```python
from build123d import *

# Parameters (mm, degrees)
SKETCH_1_W                   = 100
SKETCH_1_H                   = 100
EXTRUDE_1_DEPTH              = 5
CUT_EXTRUDE_1_REACH          = 72.887
SKETCH_2_W                   = 12.5
SKETCH_2_H                   = 22.4
HOLE_WIZARD_M2_3_D           = 2.4
HOLE_WIZARD_M2_3_CBORE_D     = 4.4
HOLE_WIZARD_M2_3_CBORE_DEPTH = 2
SKETCH_9_W                   = 25
SKETCH_9_H                   = 6.5
SKETCH_9_W_2                 = 6.5
SKETCH_9_H_2                 = 42.2
EXTRUDE_4_DEPTH              = 20
HOLE_WIZARD_M2_4_D           = 2.4
HOLE_WIZARD_M2_4_CBORE_D     = 4.4
HOLE_WIZARD_M2_4_CBORE_DEPTH = 2
SKETCH_12_W                  = 42
SKETCH_12_H                  = 5
CUT_EXTRUDE_2_DEPTH          = 10
CUT_EXTRUDE_3_DEPTH          = 91.444513377


with BuildPart() as part:
    # 草图1 → 凸台-拉伸1 (new body)
    with BuildSketch(Plane(origin=(0, 0, 0), x_dir=(1, 0, 0), z_dir=(0, 1, 0))):
        Rectangle(SKETCH_1_W, SKETCH_1_H)
    extrude(amount=EXTRUDE_1_DEPTH)

    # 草图2 → 切除-拉伸1 (cut, up to next)
    with BuildSketch(Plane(origin=(0, 5, 0), x_dir=(1, 0, 0), z_dir=(0, 1, 0)), mode=Mode.PRIVATE) as cut_extrude_1_sk1:
        with Locations((-43.75, 32.3)):
            Rectangle(SKETCH_2_W, SKETCH_2_H)
    cut_extrude_1_tool1 = extrude(cut_extrude_1_sk1.sketch, amount=-CUT_EXTRUDE_1_REACH, mode=Mode.PRIVATE) & part.part
    # 草图2 → 切除-拉伸1 (cut, up to next)
    with BuildSketch(Plane(origin=(0, 5, 0), x_dir=(1, 0, 0), z_dir=(0, 1, 0)), mode=Mode.PRIVATE) as cut_extrude_1_sk2:
        with Locations((43.75, 32.3)):
            Rectangle(SKETCH_2_W, SKETCH_2_H)
    cut_extrude_1_tool2 = extrude(cut_extrude_1_sk2.sketch, amount=-CUT_EXTRUDE_1_REACH, mode=Mode.PRIVATE) & part.part
    # 草图2 → 切除-拉伸1 (cut, up to next)
    with BuildSketch(Plane(origin=(0, 5, 0), x_dir=(1, 0, 0), z_dir=(0, 1, 0)), mode=Mode.PRIVATE) as cut_extrude_1_sk3:
        with Locations((43.75, -32.3)):
            Rectangle(SKETCH_2_W, SKETCH_2_H)
    cut_extrude_1_tool3 = extrude(cut_extrude_1_sk3.sketch, amount=-CUT_EXTRUDE_1_REACH, mode=Mode.PRIVATE) & part.part
    # 草图2 → 切除-拉伸1 (cut, up to next)
    with BuildSketch(Plane(origin=(0, 5, 0), x_dir=(1, 0, 0), z_dir=(0, 1, 0)), mode=Mode.PRIVATE) as cut_extrude_1_sk4:
        with Locations((-43.75, -32.3)):
            Rectangle(SKETCH_2_W, SKETCH_2_H)
    cut_extrude_1_tool4 = extrude(cut_extrude_1_sk4.sketch, amount=-CUT_EXTRUDE_1_REACH, mode=Mode.PRIVATE) & part.part
    add(cut_extrude_1_tool1.solids().sort_by_distance((-43.75, 5, -32.3))[0], mode=Mode.SUBTRACT)
    add(cut_extrude_1_tool2.solids().sort_by_distance((43.75, 5, -32.3))[0], mode=Mode.SUBTRACT)
    add(cut_extrude_1_tool3.solids().sort_by_distance((43.75, 5, 32.3))[0], mode=Mode.SUBTRACT)
    add(cut_extrude_1_tool4.solids().sort_by_distance((-43.75, 5, 32.3))[0], mode=Mode.SUBTRACT)

    # M2 凹头盖螺钉的柱形沉头孔3 (through all)
    with Locations(Plane(origin=(-43.75, 5, -46.15), x_dir=(0, 0, 1), z_dir=(0, 1, 0))):
        with Locations((0, 0), (0, 87.5), (27.7, 87.5), (27.7, 0), (64.6, 0), (92.3, 0), (64.6, 87.5), (92.3, 87.5)):
            CounterBoreHole(HOLE_WIZARD_M2_3_D / 2, HOLE_WIZARD_M2_3_CBORE_D / 2, HOLE_WIZARD_M2_3_CBORE_DEPTH)

    # 草图9 → 凸台-拉伸4 (add)
    with BuildSketch(Plane(origin=(0, 5, 0), x_dir=(1, 0, 0), z_dir=(0, 1, 0))):
        with Locations((0, 46.75)):
            Rectangle(SKETCH_9_W, SKETCH_9_H)
        with Locations((0, -46.75)):
            Rectangle(SKETCH_9_W, SKETCH_9_H)
        with Locations((-34.25, 0)):
            Rectangle(SKETCH_9_W_2, SKETCH_9_H_2)
        with Locations((34.25, 0)):
            Rectangle(SKETCH_9_W_2, SKETCH_9_H_2)
    extrude(amount=EXTRUDE_4_DEPTH)

    # M2 凹头盖螺钉的柱形沉头孔4 (through all)
    with Locations(Plane(origin=(-17, 5, -25), x_dir=(0, 0, 1), z_dir=(0, 1, 0))):
        with Locations((0, 0), (0, 34), (50, 0), (50, 34)):
            CounterBoreHole(HOLE_WIZARD_M2_4_D / 2, HOLE_WIZARD_M2_4_CBORE_D / 2, HOLE_WIZARD_M2_4_CBORE_DEPTH)

    # 草图12 → 切除-拉伸2 (cut)
    with BuildSketch(Plane(origin=(0, 5, 0), x_dir=(1, 0, 0), z_dir=(0, 1, 0))):
        with Locations((0, 36.5)):
            Rectangle(SKETCH_12_W, SKETCH_12_H)
        with Locations((0, -36.5)):
            Rectangle(SKETCH_12_W, SKETCH_12_H)
    extrude(amount=-CUT_EXTRUDE_2_DEPTH, mode=Mode.SUBTRACT)

    # 草图15 → 切除-拉伸3 (cut, through all)
    with BuildSketch(Plane.XY.offset(21.1)):
        Polygon((-37.5, 25), (-37.5, 22), (-35.5, 22), align=None)
        Polygon((-31, 25), (-31, 22), (-33, 22), align=None)
        Polygon((37.5, 25), (37.5, 22), (35.5, 22), align=None)
        Polygon((31, 22), (33, 22), (31, 25), align=None)
    extrude(amount=-CUT_EXTRUDE_3_DEPTH, mode=Mode.SUBTRACT)


solid = part.part
```
CAD build for the part. Positions are in the model's coordinates, mm. A direction names the side the tool comes from. Coordinates: 2 decimals unless noted, no trailing zeros. Order: outer loops, then holes, each group sorted by start corner. A loop starts at its lowest first (then second) coordinate and runs counter-clockwise, first axis right, second up. Notation, with made-up numbers: (88.25, -17.75) - (143.25, -17.75) arc R18 cw to (143.25, 14.25) - close; hole circle Ø1 at (63, -1). An arc over 180 degrees is marked (long way). Answer in a Markdown table with one row per item.
1. Drill centre lines: L1, parallel to X at y = 4.05, z = -46.15; L2, parallel to X at y = 1.35, z = -18.45; L3, parallel to Z at x = -19.5, y = 4. Where is each one in solid material? Low to high. Write a range as from..to.
Answer:
| item | result |
|---|---|
| L1 | -50..-45.95, -41.55..41.55, 45.95..50 |
| L2 | -50..-44.95, -42.55..42.55, 44.95..50 |
| L3 | -50..-39, -34..34, 39..50 |
2. 3-axis set-ups, long thin cutter, end or side, ignore diameter. For faces 1 (the face through (12.5, 15, -47)), 2 (the face through (-45.7, 4.01, -45.13)), 3 (the face through (0, 15, 43.5)): which of +Z, -Z, +X, -X, +Y, -Y reach the whole face in a straight line?
Answer:
| item | result |
|---|---|
| face 1 | +Z, -Z, +X, +Y |
| face 2 | +Y |
| face 3 | +X, -X, +Y |
3. Slice it at A-A, the plane x = 9.5. List the corners of the cut face in (y, z), then the cut area to 3 significant figures.
Answer:
| item | result |
|---|---|
| outline | (0, -50) - (25, -50) - (25, -43.5) - (5, -43.5) - (5, -39) - (0, -39) - close; (0, -34) - (5, -34) - (5, 34) - (0, 34) - close; (0, 39) - (5, 39) - (5, 43.5) - (25, 43.5) - (25, 50) - (0, 50) - close |
| area | 710 mm² |
4. Pull direction X, two halves, no side cores. Call faces 4 (the face through (-37.5, 3, 32)), 5 (the face through (50, 2, 0)), 6 (the face through (16, 3, -24)), 7 (the face through (-1, 10, -50)): +X half, -X half, draft (parallel to the pull), parting line (faces both ways), or undercut.
Answer:
| item | result |
|---|---|
| face 4 | -X half |
| face 5 | +X half |
| face 6 | undercut |
| face 7 | draft |
5. Slice it at C-C, the plane x = -17. List the corners of the cut face in (y, z), then the cut area to 3 significant figures.
Answer:
| item | result |
|---|---|
| outline | (0, -50) - (5, -50) - (5, -39) - (0, -39) - close; (0, -34) - (5, -34) - (5, -27.2) - (3, -27.2) - (3, -26.2) - (0, -26.2) - close; (0, -23.8) - (3, -23.8) - (3, -22.8) - (5, -22.8) - (5, 22.8) - (3, 22.8) - (3, 23.8) - (0, 23.8) - close; (0, 26.2) - (3, 26.2) - (3, 27.2) - (5, 27.2) - (5, 34) - (0, 34) - close; (0, 39) - (5, 39) - (5, 50) - (0, 50) - close |
| area | 418 mm² |
6. Flat gauge pins, fed straight in: P1, Ø5, axis at x = -43.5, z = 46, coming from the +Y side; P2, Ø2, axis at y = 10.5, z = 46, coming from the +X side; P3, Ø3.5, axis at x = 43.75, z = 18.45, coming from the -Y side; P4, Ø8.5, axis at y = 15, z = -7.5, coming from the +X side. Where does each tip first touch, or does it go through?
Answer:
| item | result |
|---|---|
| P1 | y = 5 |
| P2 | x = 12.5 |
| P3 | y = 0 |
| P4 | x = 37.5 |
7. Slice it at D-D, the plane z = 46.15. List the corners of the cut face in (x, y).
Answer:
| item | result |
|---|---|
| outline | (-50, 0) - (-44.95, 0) - (-44.95, 3) - (-45.95, 3) - (-45.95, 5) - (-50, 5) - close; (-42.55, 0) - (42.55, 0) - (42.55, 3) - (41.55, 3) - (41.55, 5) - (12.5, 5) - (12.5, 25) - (-12.5, 25) - (-12.5, 5) - (-41.55, 5) - (-41.55, 3) - (-42.55, 3) - close; (44.95, 0) - (50, 0) - (50, 5) - (45.95, 5) - (45.95, 3) - (44.95, 3) - close |
8. Slice it at B-B, the plane z = -25. List the corners of the cut face in (x, y).
Answer:
| item | result |
|---|---|
| outline | (-37.5, 0) - (-18.2, 0) - (-18.2, 3) - (-19.2, 3) - (-19.2, 5) - (-37.5, 5) - close; (-15.8, 0) - (15.8, 0) - (15.8, 3) - (14.8, 3) - (14.8, 5) - (-14.8, 5) - (-14.8, 3) - (-15.8, 3) - close; (18.2, 0) - (37.5, 0) - (37.5, 5) - (19.2, 5) - (19.2, 3) - (18.2, 3) - close |
